```python
from build123d import *

# Parameters (mm, degrees)
F0_W     = 88.1328396499
F0_H     = 62.7489611506
F1_DEPTH = 41.656
F3_DEPTH = 2514.6
F4_DEPTH = 25.4
F6_DEPTH = 25.4
F7_R     = 4.0308463813
F8_R     = 3.5011356281
F9_DEPTH = 2514.6


with BuildPart() as f1:
    # F0 (on Top) → F1 (new body)
    with BuildSketch(Plane.XY):
        with Locations((4.3660271913, -7.5136311352)):
            Rectangle(F0_W, F0_H)
    extrude(amount=F1_DEPTH)

    # F2 (on face) → F3 (cut)
    with BuildSketch(Plane.XZ.offset(38.8881117105)):
        with BuildLine():
            Line((34.01440382, 41.656), (-21.2209261954, 41.656))
            ThreePointArc((-21.2209261954, 41.656), (6.3967388123, 26.2462017045), (34.01440382, 41.656))
        make_face()
    extrude(amount=-F3_DEPTH, mode=Mode.SUBTRACT)

    # F2 (on face) → F4 (join)
    with BuildSketch(Plane.XZ.offset(38.8881117105)):
        with BuildLine():
            ThreePointArc((34.01440382, 41.656), (6.3967388123, 26.2462017045), (-21.2209261954, 41.656))
            Line((-21.2209261954, 41.656), (-28.734555468, 41.656))
            ThreePointArc((-28.734555468, 41.656), (4.6706357971, 19.5296360838), (38.0758270621, 41.656))
            Line((38.0758270621, 41.656), (34.01440382, 41.656))
        make_face()
    extrude(amount=F4_DEPTH)

    # F5 (on face) → F6 (join)
    with BuildSketch(Plane(origin=(0, 23.8608494401, 0), x_dir=(-1, 0, 0), z_dir=(0, 1, 0))):
        with BuildLine():
            Line((-34.01440382, 41.656), (-38.1010249257, 41.656))
            ThreePointArc((-38.1010249257, 41.656), (-5.3521022201, 20.4356830154), (27.3968204856, 41.656))
            Line((27.3968204856, 41.656), (21.2209261954, 41.656))
            ThreePointArc((21.2209261954, 41.656), (-6.3967388123, 26.2462017045), (-34.01440382, 41.656))
        make_face()
    extrude(amount=F6_DEPTH)

    # F7 (on face) + F8 (on face) → F9 (cut)
    with BuildSketch(Plane.XY.offset(41.656)):
        with Locations((-33.8113345206, -2.9445304535)):
            Circle(F7_R)
    with BuildSketch(Plane.XY.offset(41.656)):
        with Locations((41.7311042547, 0)):
            Circle(F8_R)
    extrude(amount=-F9_DEPTH, mode=Mode.SUBTRACT)


solid = f1.part
```
Here's how the part is built. I have some questions about the finished solid (model axes, mm). A direction names the side the tool comes from. Give positions to 0.01 mm unless a question says otherwise; leave off trailing zeros. Write each loop counter-clockwise with the first axis right and the second up, starting at its lowest first coordinate (ties: lowest second). Pieces come first, ordered by that corner, then holes. Notation, with made-up numbers: (-12, 32.5) -> (33, 32.5) arc R8 ccw to (33, 46.5) -> close; hole circle Ø7 at (57.5, 85.5). An arc over 180 degrees is marked (long way). Write each question's results on one line, items separated by ' | '.
Item 1: Suppose I cut it at A-A on z = 27.5. Write out the boundary of the cut face in (x, y), plus the area to 3 significant figures.
Output:
outline: (-39.7, -38.89) -> (-18.02, -38.89) -> (-18.02, -64.29) -> (-2.54, -64.29) -> (-2.54, 49.26) -> (-16.03, 49.26) -> (-16.03, 23.86) -> (-39.7, 23.86) -> close; (15.33, -64.29) -> (27.36, -64.29) -> (27.36, -38.89) -> (48.43, -38.89) -> (48.43, 23.86) -> (26.73, 23.86) -> (26.73, 49.26) -> (15.33, 49.26) -> close; hole circle Ø8.06 at (-33.81, -2.94); hole circle Ø7 at (41.73, 0) | area: 5,650 mm^2
Item 2: Suppose I cut it at C-C on y = -23.5. Write out the boundary of the cut face in (x, z), plus the area to 3 significant figures.
Output:
outline: (-39.7, 0) -> (48.43, 0) -> (48.43, 41.66) -> (34.01, 41.66) arc R32.45 cw to (-21.22, 41.66) -> (-39.7, 41.66) -> close | area: 3,070 mm^2
Item 3: If I drill on L1, parallel to Y at x = 33.5, z = 9.5; L2, parallel to Y at x = -35, z = 11; L3, parallel to X at y = 27, z = 39.5, over which ranges is the centre line in solid material (lowest first)?
Output:
L1: y = -38.89 to 23.86 | L2: y = -38.89 to -6.8, 0.91 to 23.86 | L3: x = -26.34 to -19.77, 32.56 to 37.05
Item 4: On a 3-axis mill with a long thin cutter (end or side, diameter ignored), from which of +Z, -Z, +X, -X, +Y, -Y can I reach the whole of each face in a straight line? I mean faces 1 (the face through (5.93, 36.38, 20.44)), 2 (the face through (4, -38.888, 16)), 3 (the face through (4, -7, 0)). Say none if no direction works.
Output:
face 1: -Z, +Y | face 2: -Z, -Y | face 3: -Z, +X, -X, +Y, -Y
Item 5: Suppose I cut it at B-B on x = 3.5. Write out the boundary of the cut face in (y, z).
Output:
outline: (-64.29, 19.55) -> (-38.89, 19.55) -> (-38.89, 0) -> (23.86, 0) -> (23.86, 20.48) -> (49.26, 20.48) -> (49.26, 26.38) -> (-64.29, 26.38) -> close
Item 6: Suppose I cut it at D-D on z = 35. Write out the boundary of the cut face in (x, y).
Output:
outline: (-39.7, -38.89) -> (-25.05, -38.89) -> (-25.05, -64.29) -> (-15.77, -64.29) -> (-15.77, 49.26) -> (-23.51, 49.26) -> (-23.51, 23.86) -> (-39.7, 23.86) -> close; (28.57, -64.29) -> (34.39, -64.29) -> (34.39, -38.89) -> (48.43, -38.89) -> (48.43, 23.86) -> (34.21, 23.86) -> (34.21, 49.26) -> (28.57, 49.26) -> close; hole circle Ø8.06 at (-33.81, -2.94); hole circle Ø7 at (41.73, 0)
Item 7: We'd pull the mould along X, two halves only. Please class faces 4 (the face through (-37.84, -2.77, 21.12)), 5 (the face through (-0.4, -64.288, 26.5)), 6 (the face through (4.076, -51.41, 19.535)): pulls with the +X half, pulls with the -X half, needs draft (parallel to the pull), parting line crosses it, or undercut.
Output:
face 4: undercut | face 5: needs draft | face 6: parting line crosses it
Item 8: For pin 1 Ø5 at (x, y) = (-25.5, 20.5) entering from -Z; pin 2 Ø5 at (x, z) = (11, 10.5) entering from -Y, each with a flat end and sliding along its axis, tell me the tip position at first contact or that it passes through.
Output:
pin 1: stops at z = 0 | pin 2: stops at y = -38.89
